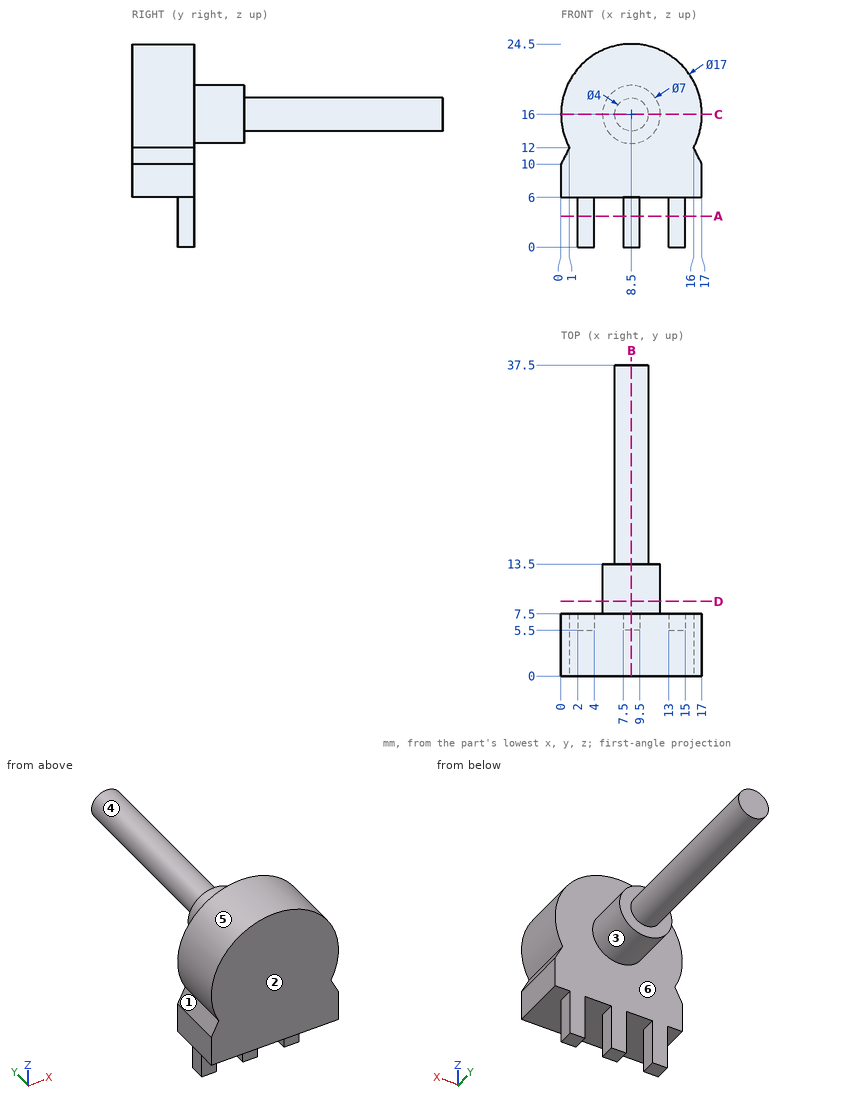
Could you check a few things on this drawing? It's one solid part, dimensions in mm from its lowest x, y, z. A direction names the side the tool comes from. Coordinates: 2 decimals unless noted, no trailing zeros. Order: outer loops, then holes, each group sorted by start corner. A loop starts at its lowest first (then second) coordinate and runs counter-clockwise, first axis right, second up.
1) Which directions (+Z, -Z, +X, -X, +Y, -Y) give clear straight access to the entire face, cutting with the end or side of a thin tool? Please do the marked faces 1, 2 and 3.
2) Imagine slicing it at D-D on y = 9. List the corners of the cut face in (x, z) for me.
3) We'd pull the mould along Z, two halves only. Please class the marked faces 4, 5 and 6: +Z half, -Z half, draft (parallel to the pull), parting line (faces both ways), or undercut.
4) Imagine slicing it at A-A on z = 3.75. List the corners of the cut face in (x, y) for me, and give its area (3 significant figures).
5) Will these pins go through, and if not, where does the flat tip stop? pin 1 (2 mm diameter, centred on y = 7, z = 2.5, fed in from -X); pin 2 (0.6 mm diameter, centred on x = 3, z = 3, fed in from -Y); pin 3 (1 mm diameter, centred on y = 6.5, z = 2.5, fed in from +X).
6) Imagine slicing it at C-C on z = 16. List the corners of the cut face in (x, y) for me.
7) Imagine slicing it at B-B on x = 8.5. List the corners of the cut face in (y, z) for me, and give its area (3 significant figures).
8) I need wall thicknesses on line 1 (X direction, y = 7, z = 3.25); line 2 (Y direction, x = 7.25, z = 10.75); line 3 (Y direction, x = 8.5, z = 13.25). Which ranges of each line are inside material? Lowest first, please.
Response values:
1. face 1: -X, +Y, -Y
1. face 2: +Z, -Z, +X, -X, -Y
1. face 3: +Y
2. outline: circle Ø7 at (8.5, 16)
3. face 4: parting line
3. face 5: undercut
3. face 6: draft
4. outline: (2, 5.5) - (4, 5.5) - (4, 7.5) - (2, 7.5) - close; (7.5, 5.5) - (9.5, 5.5) - (9.5, 7.5) - (7.5, 7.5) - close; (13, 5.5) - (15, 5.5) - (15, 7.5) - (13, 7.5) - close
4. area: 12.0 mm2
5. pin 1: stops at x = 2
5. pin 2: stops at y = 5.5
5. pin 3: stops at x = 15
6. outline: (0, 0) - (17, 0) - (17, 7.5) - (12, 7.5) - (12, 13.5) - (10.5, 13.5) - (10.5, 37.5) - (6.5, 37.5) - (6.5, 13.5) - (5, 13.5) - (5, 7.5) - (0, 7.5) - close
7. outline: (0, 6) - (5.5, 6) - (5.5, 0) - (7.5, 0) - (7.5, 12.5) - (13.5, 12.5) - (13.5, 14) - (37.5, 14) - (37.5, 18) - (13.5, 18) - (13.5, 19.5) - (7.5, 19.5) - (7.5, 24.5) - (0, 24.5) - close
7. area: 289 mm2
8. line 1: x = 2 to 4, 7.5 to 9.5, 13 to 15
8. line 2: y = 0 to 7.5
8. line 3: y = 0 to 13.5
